CAD build for the part. Positions are in the model's coordinates, mm. A direction names the side the tool comes from. Round coordinates to 2 decimals unless told otherwise and drop trailing zeros. Order: outer loops, then holes, each group sorted by start corner. A loop starts at its lowest first (then second) coordinate and runs counter-clockwise, first axis right, second up. Notation, with made-up numbers: M 39.25,88 L 68.25,88 A28 ccw 68.25,126 Z; hole C 16.25,-34.75 d4. An arc over 180 degrees is marked long. Answer as a JSON object with one key per item and string values.
```python
from build123d import *

# Parameters (mm, degrees)
SKETCH1_R        = 9.74
SKETCH1_R_2      = 2.57
MOUNTBODY_DEPTH  = 4.1
SKETCH2_R        = 3.5
SKETCH2_R_2      = 1.67
CAP_DEPTH        = 0.2
SKETCH3_R        = 0.75
SCREWHOLES_DEPTH = 15.371680486


with BuildPart() as part:
    # Sketch1 → MountBody (new body)
    with BuildSketch(Plane(origin=(0, 0, 0), x_dir=(1, 0, 0), z_dir=(0, 1, 0))):
        with Locations(Location((0, 0, 0), (0, 0, 270))):
            Circle(SKETCH1_R)
        with Locations(Location((0, 0, 0), (0, 0, 270))):
            Circle(SKETCH1_R_2, mode=Mode.SUBTRACT)
    extrude(amount=MOUNTBODY_DEPTH)

    # Sketch2 → Cap (add)
    with BuildSketch(Plane(origin=(0, 4.1, 0), x_dir=(1, 0, 0), z_dir=(0, 1, 0))):
        with Locations(Location((0, 0, 0), (0, 0, 270))):
            Circle(SKETCH2_R)
        with Locations(Location((0, 0, 0), (0, 0, 270))):
            Circle(SKETCH2_R_2, mode=Mode.SUBTRACT)
    extrude(amount=CAP_DEPTH)

    # Sketch3 → ScrewHoles (cut, through all)
    with BuildSketch(Plane(origin=(0, 4.1, 0), x_dir=(1, 0, 0), z_dir=(0, 1, 0))):
        with Locations(Location((6, 0, 0), (0, 0, 270))):
            Circle(SKETCH3_R)
        with Locations(Location((4.242640687, -4.242640687, 0), (0, 0, 270))):
            Circle(SKETCH3_R)
        with Locations(Location((0, -6, 0), (0, 0, 270))):
            Circle(SKETCH3_R)
        with Locations(Location((-4.242640687, -4.242640687, 0), (0, 0, 270))):
            Circle(SKETCH3_R)
        with Locations(Location((-6, 0, 0), (0, 0, 270))):
            Circle(SKETCH3_R)
        with Locations(Location((-4.242640687, 4.242640687, 0), (0, 0, 270))):
            Circle(SKETCH3_R)
        with Locations(Location((0, 6, 0), (0, 0, 270))):
            Circle(SKETCH3_R)
        with Locations(Location((4.242640687, 4.242640687, 0), (0, 0, 270))):
            Circle(SKETCH3_R)
    extrude(amount=-SCREWHOLES_DEPTH, mode=Mode.SUBTRACT)


solid = part.part
```
Item 1: Saw through at A-A on z = 0. List the corners of the cut face in (x, y).
Worked answers:
{"outline": "M -9.74,0 L -6.75,0 L -6.75,4.1 L -9.74,4.1 Z; M -5.25,0 L -2.57,0 L -2.57,4.1 L -1.67,4.1 L -1.67,4.3 L -3.5,4.3 L -3.5,4.1 L -5.25,4.1 Z; M 1.67,4.1 L 2.57,4.1 L 2.57,0 L 5.25,0 L 5.25,4.1 L 3.5,4.1 L 3.5,4.3 L 1.67,4.3 Z; M 6.75,0 L 9.74,0 L 9.74,4.1 L 6.75,4.1 Z"}
Item 2: Saw through at D-D on x = 6. List the corners of the cut face in (y, z).
Worked answers:
{"outline": "M 0,-7.67 L 4.1,-7.67 L 4.1,-0.75 L 0,-0.75 Z; M 0,0.75 L 4.1,0.75 L 4.1,7.67 L 0,7.67 Z"}
Item 3: Wall check: line 1 along X through (y, z) = (2.95, 0); line 2 along X through (y, z) = (2.85, 4.75); line 3 along X through (y, z) = (0.6, -4). Give the ranges that are in metal, low to high. Write a range as [from, to].
Worked answers:
{"line 1": "x = [-9.74, -6.75], [-5.25, -2.57], [2.57, 5.25], [6.75, 9.74]", "line 2": "x = [-8.5, -4.79], [-3.69, 3.69], [4.79, 8.5]", "line 3": "x = [-8.88, -4.95], [-3.53, 3.53], [4.95, 8.88]"}
Item 4: 3-axis set-ups, long thin cutter, end or side, ignore diameter. For faces 4 (the cylindrical face through (-4.975, 2.079, 4.08)), 5 (the flat face through (0, 4.1, 2)): which of +Z, -Z, +X, -X, +Y, -Y reach the whole face in a straight line?
Worked answers:
{"face 4": "+Y, -Y", "face 5": "-Y"}
Item 5: Two-plate mould, pull along Z, no slides. Class faces 1 (the flat face through (0, 4.1, 4)), 2 (the cylindrical face through (-4.975, 2.079, -4.405)), 3 (the cylindrical face through (2.9, 2, 9.3)): released by +Z, released by -Z, zero draft, split by the parting line, or undercut.
Worked answers:
{"face 1": "zero draft", "face 2": "undercut", "face 3": "split by the parting line"}
Item 6: Saw through at B-B on x = 0. List the corners of the cut face in (y, z).
Worked answers:
{"outline": "M 0,-9.74 L 4.1,-9.74 L 4.1,-6.75 L 0,-6.75 Z; M 0,-5.25 L 4.1,-5.25 L 4.1,-3.5 L 4.3,-3.5 L 4.3,-1.67 L 4.1,-1.67 L 4.1,-2.57 L 0,-2.57 Z; M 0,2.57 L 4.1,2.57 L 4.1,1.67 L 4.3,1.67 L 4.3,3.5 L 4.1,3.5 L 4.1,5.25 L 0,5.25 Z; M 0,6.75 L 4.1,6.75 L 4.1,9.74 L 0,9.74 Z"}
Item 7: Drop flat-ended pins along their axis: pin 1 Ø2 at (x, y) = (6, 1.5) entering from -Z; pin 2 Ø1.5 at (x, z) = (-1, -1) entering from -Y; pin 3 Ø2.5 at (x, z) = (-4.24, 4.24) entering from +Y. Give the stop position or say it passes through.
Worked answers:
{"pin 1": "stops at z = -8.36", "pin 2": "stops at y = 4.1", "pin 3": "stops at y = 4.1"}
Item 8: Saw through at C-C on z = 6. List the corners of the cut face in (x, y).
Worked answers:
{"outline": "M -7.67,0 L -0.75,0 L -0.75,4.1 L -7.67,4.1 Z; M 0.75,0 L 7.67,0 L 7.67,4.1 L 0.75,4.1 Z"}
